from build123d import *

# Parameters (mm, degrees)
SKETCH2_W           = 1500
SKETCH2_H           = 1500
BOSS_EXTRUDE1_DEPTH = 10
BOSS_EXTRUDE2_DEPTH = 110
BOSS_EXTRUDE3_DEPTH = 110


with BuildPart() as part:
    # Sketch2 → Boss-Extrude1 (new body)
    with BuildSketch(Plane(origin=(0, 0, 0), x_dir=(1, 0, 0), z_dir=(0, 1, 0))):
        Rectangle(SKETCH2_W, SKETCH2_H)
    extrude(amount=BOSS_EXTRUDE1_DEPTH)

    # Sketch3 → Boss-Extrude2 (add)
    with BuildSketch(Plane(origin=(0, 10, 0), x_dir=(1, 0, 0), z_dir=(0, 1, 0))):
        with BuildLine():
            ThreePointArc((750, -600), (-204.594154602, -204.594154602), (-600, 750))
            Line((-600, 750), (-620, 750))
            ThreePointArc((-620, 750), (-218.736290226, -218.736290226), (750, -620))
            Line((750, -620), (750, -600))
        make_face()
        with BuildLine():
            Line((620, 750), (600, 750))
            ThreePointArc((600, 750), (643.933982822, 643.933982822), (750, 600))
            Line((750, 600), (750, 620))
            ThreePointArc((750, 620), (658.076118446, 658.076118446), (620, 750))
        make_face()
    extrude(amount=BOSS_EXTRUDE2_DEPTH)

    # Sketch4 → Boss-Extrude3 (add)
    with BuildSketch(Plane(origin=(0, 10, 0), x_dir=(1, 0, 0), z_dir=(0, 1, 0))):
        Polygon((545.174998191, 531.032862568), (651.241015369, 637.098879746), (637.098879746, 651.241015369), (531.032862568, 545.174998191), align=None)
    extrude(amount=BOSS_EXTRUDE3_DEPTH)


solid = part.part
Source: CAD feature listing. Evaluate the final solid. Frame: model axes, mm. A direction names the side the tool comes from. Coordinates: 2 decimals unless noted, no trailing zeros. Loops run counter-clockwise (first coordinate to the right, second up) from the corner with the lowest first, then second, coordinate; pieces in that order, holes last. Notation, with made-up numbers: (54, 67.25) - (78, 67.25) arc R15 ccw to (78, 95.25) - close; hole circle Ø4 at (-9, 29). An arc over 180 degrees is marked (long way). One line per item, written item: value. Start each with the question number.
1. Section D-D (z = 640). Return the cut outline in (x, y).
2. Section A-A (y = 82.5). Return the cut outline in (x, z) (3 decimals), and give its area (3 significant figures).
3. Mould query, pull axis X, two halves, no side actions, for faces 5 (the cylindrical face through (609.3, 64.2, -698)), 6 (the flat face through (216, 10, -234)), 7 (the flat face through (-4, 2, -750)), 8 (the flat face through (750, 2, 4)). Classes: pulls with the +X half, pulls with the -X half, needs draft (parallel to the pull), parting line crosses it, or undercut.
4. Section C-C (x = 412.5). Return the cut outline in (y, z).
5. Contact query for flat-ended pins moving along their axis: P1, Ø5, axis at x = 321, y = 27.5, coming from the +Z side; P2, Ø5, axis at x = -51.5, y = 43.5, coming from the +Z side; P3, Ø4, axis at x = 101, y = 36, coming from the -Z side. Output: stop coordinate, or through.
6. Section B-B (z = 104.5). Return the cut outline in (x, y), and give its area (3 significant figures).
7. Set-up query: faces 1 (the flat face through (584.81, 64.23, -598.95)), 2 (the flat face through (699, 10, -700)), 3 (the cylindrical face through (-229.329, 64.23, 208.026)), 4 (the flat face through (-10, 0, -10)). Return all of +Z, -Z, +X, -X, +Y, -Y with unobstructed straight access to the full face (end or side cutting, diameter ignored); none if empty.
8. Ray query, L1, parallel to Y at x = 13, z = -440.5; L2, parallel to X at y = 18.5, z = -541.5; L3, parallel to X at y = 70.5, z = -541. Return the intervals inside material, ascending.
Verdict:
1. outline: (-750, 0) - (750, 0) - (750, 10) - (-750, 10) - close
2. outline: (-620, -750) - (-600, -750) arc R1350 cw to (750, 600) - (750, 620) arc R1370 ccw to start; (531.033, -545.175) - (637.099, -651.241) arc R150 ccw to (600, -750) - (620, -750) arc R130 cw to (750, -620) - (750, -600) arc R150 ccw to (651.241, -637.099) - (545.175, -531.033) - close
2. area: 50,100 mm2
3. face 5: undercut
3. face 6: undercut
3. face 7: needs draft
3. face 8: pulls with the +X half
4. outline: (0, -750) - (10, -750) - (10, 557.13) - (120, 557.13) - (120, 577.78) - (10, 577.78) - (10, 750) - (0, 750) - close
5. P1: stops at z = 551.92
5. P2: stops at z = 362.88
5. P3: stops at z = 432.67
6. outline: (-750, 0) - (750, 0) - (750, 10) - (-295.15, 10) - (-295.15, 120) - (-320.85, 120) - (-320.85, 10) - (-750, 10) - close
6. area: 17,800 mm2
7. face 1: +Y
7. face 2: -Z, +X, +Y
7. face 3: +Z, -X, +Y
7. face 4: +Z, -Z, +X, -X, -Y
8. L1: y = 0 to 10
8. L2: x = -604.04 to -583.8, 534.71 to 555.64
8. L3: x = -603.96 to -583.72, 535.21 to 555.14
